from build123d import *

# Parameters (mm, degrees)
BOSS_EXTRUDE1_DEPTH      = 9.9
BOSS_EXTRUDE1_DEPTH_BACK = 9.9
SKETCH1_W                = 7.5
SKETCH1_H                = 7.5
SKETCH1_R                = 1.6
BOSS_EXTRUDE2_DEPTH      = 19.8


with BuildPart() as part:
    # Sketch1 → Boss-Extrude1 (new, two sides: drawn at the far end of the back side and taken through both)
    with BuildSketch(Plane.XY.offset(-BOSS_EXTRUDE1_DEPTH_BACK)):
        Rectangle(SKETCH1_W, SKETCH1_H)
        Circle(SKETCH1_R, mode=Mode.SUBTRACT)
    extrude(amount=BOSS_EXTRUDE1_DEPTH + BOSS_EXTRUDE1_DEPTH_BACK)

    # Sketch2 → Boss-Extrude2 (add)
    with BuildSketch(Plane.XY.offset(9.9)):
        Polygon((3.75, 3.75), (6.75, 6.75), (8.75, 6.75), (7.595299462, 8.75), (1.25, 8.75), (-3.75, 3.75), align=None)
    extrude(amount=-BOSS_EXTRUDE2_DEPTH)


solid = part.part
Work out the finished part from the listing and answer in its coordinate system (mm). A direction names the side the tool comes from. Round coordinates to 2 decimals unless told otherwise and drop trailing zeros. Loops run counter-clockwise (first coordinate to the right, second up) from the corner with the lowest first, then second, coordinate; pieces in that order, holes last. Notation, with made-up numbers: M -39.5,-20.75 L 13.5,-20.75 A15 cw 13.5,1.25 Z; hole C -39,33.25 d4. An arc over 180 degrees is marked long. One line per question, with ' | ' between items. Start each with the question number.
(1) A tool of negligible diameter and unlimited length cuts with its end or side. For faces 4 (the face through (1, 3, -9.9)), 5 (the face through (8, 6.75, 0)), from which of +Z, -Z, +X, -X, +Y, -Y can it reach the whole face along a straight path? Write none if from no direction.
(2) Find the intervals of material crossed by line 1 (X direction, y = -2.75, z = 5.75); line 2 (Y direction, x = 0, z = 0.5); line 3 (X direction, y = -1, z = -4.75), in increasing order.
(3) A cutting plane is placed at D-D on y = 4. Write down the section's boundary in (x, z), plus the area to 4 significant figures.
(4) A cutting plane is placed at A-A on x = 0. Write down the section's boundary in (y, z).
(5) A cutting plane is placed at C-C on z = -2. Write down the section's boundary in (x, y).
(6) Flat-ended cylindrical pins translate along their axes: pin 1 Ø4 at (y, z) = (0, -1) entering from +X; pin 2 Ø1.5 at (x, z) = (6, -1.5) entering from -Y; pin 3 Ø1 at (x, z) = (8, 1.5) entering from -Y. Find the tip coordinate at first contact, or state that the pin passes through.
(7) A cutting plane is placed at B-B on y = 0. Write down the section's boundary in (x, z), plus the area to 3 significant figures.
(8) For a pull along Y with two mould halves and no side action, classify faces 1 (the face through (8.2, 7.7, 0.1)), 2 (the face through (-3.75, 0, 0)), 3 (the face through (-1.27, -0.97, -0.14)) as released by +Y, released by -Y, zero draft, split by the parting line, or undercut.
Geometry check:
1) face 4: -Z, +X, -X, +Y, -Y | face 5: +Z, -Z, +X, -Y
2) line 1: x = -3.75 to 3.75 | line 2: y = -3.75 to -1.6, 1.6 to 7.5 | line 3: x = -3.75 to -1.25, 1.25 to 3.75
3) outline: M -3.5,-9.9 L 4,-9.9 L 4,9.9 L -3.5,9.9 Z | area: 148.5 mm²
4) outline: M -3.75,-9.9 L -1.6,-9.9 L -1.6,9.9 L -3.75,9.9 Z; M 1.6,-9.9 L 7.5,-9.9 L 7.5,9.9 L 1.6,9.9 Z
5) outline: M -3.75,-3.75 L 3.75,-3.75 L 3.75,3.75 L 6.75,6.75 L 8.75,6.75 L 7.6,8.75 L 1.25,8.75 L -3.75,3.75 Z; hole C 0,0 d3.2
6) pin 1: stops at x = 3.75 | pin 2: stops at y = 5.25 | pin 3: stops at y = 6.75
7) outline: M -3.75,-9.9 L -1.6,-9.9 L -1.6,9.9 L -3.75,9.9 Z; M 1.6,-9.9 L 3.75,-9.9 L 3.75,9.9 L 1.6,9.9 Z | area: 85.1 mm²
8) face 1: released by +Y | face 2: zero draft | face 3: undercut
